```python
from build123d import *

# Parameters (mm, degrees)
SKETCH1_R           = 3.175
BOSS_EXTRUDE1_DEPTH = 25.4
SKETCH2_W           = 5.08
SKETCH2_H           = 2.9464
CUT_EXTRUDE1_DEPTH  = 9.144
BOSS_EXTRUDE2_START = 0.508
SKETCH3_R           = 3.175
BOSS_EXTRUDE2_DEPTH = 0.508
SKETCH4_R           = 2.667
SKETCH4_W           = 5.08
SKETCH4_H           = 2.921
CUT_EXTRUDE2_DEPTH  = 1.524


with BuildPart() as part:
    # Sketch1 → Boss-Extrude1 (new body)
    with BuildSketch(Plane(origin=(0, 0, 0), x_dir=(1, 0, 0), z_dir=(0, 1, 0))):
        with Locations(Location((0, 0, 0), (0, 0, 270))):
            Circle(SKETCH1_R)
    extrude(amount=BOSS_EXTRUDE1_DEPTH)

    # Sketch2 → Cut-Extrude1 (cut)
    with BuildSketch(Plane.XZ):
        Rectangle(SKETCH2_W, SKETCH2_H)
    extrude(amount=-CUT_EXTRUDE1_DEPTH, mode=Mode.SUBTRACT)

    # Sketch3 → Boss-Extrude2 (add)
    with BuildSketch(Plane.XZ.offset(BOSS_EXTRUDE2_START)):
        with Locations(Location((0, 0, 0), (0, 0, 270))):
            Circle(SKETCH3_R)
    extrude(amount=-BOSS_EXTRUDE2_DEPTH)

    # Sketch4 → Cut-Extrude2 (cut)
    with BuildSketch(Plane.XZ.offset(0.508)):
        Circle(SKETCH4_R)
        Rectangle(SKETCH4_W, SKETCH4_H)
    extrude(amount=-CUT_EXTRUDE2_DEPTH, mode=Mode.SUBTRACT)


solid = part.part
```
Build history of the part. All positions in model axes, mm. A direction names the side the tool comes from. Coordinates: 2 decimals unless noted, no trailing zeros. Order: outer loops, then holes, each group sorted by start corner. A loop starts at its lowest first (then second) coordinate and runs counter-clockwise, first axis right, second up. Notation, with made-up numbers: (-26.5, 68) -> (-14.5, 68) arc R11 ccw to (-14.5, 77) -> close; hole circle Ø8 at (-30.5, 81). An arc over 180 degrees is marked (long way). Answer in a Markdown table with one row per item. Add a question column.
Q1. Drop flat-ended pins along their axis: pin 1 (1.3 mm diameter, centred on x = 1, z = -2, fed in from -Y); pin 2 (0.9 mm diameter, centred on x = -1, z = -0.5, fed in from -Y); pin 3 (0.5 mm diameter, centred on y = 0.5, z = -1, fed in from -X); pin 4 (0.6 mm diameter, centred on y = 0, z = 1, fed in from +X). Give the stop position or say it passes through.
Q2. Mould opens along Y. For faces 3 (the face through (0, 1.016, -2)), 4 (the face through (0, 25.4, 0)) say: +Y half, -Y half, draft (parallel to the pull), parting line (faces both ways), or undercut.
Q3. Which spindle directions (+Z, -Z, +X, -X, +Y, -Y) get a long thin tool onto all of the face, cutting with end or side? Do faces 1 (the face through (2.667, 0.243, -0.012)), 2 (the face through (-2, -0.508, 2)). Say none if no direction does.
Q4. Wall check: line 1 along X through (y, z) = (3.5, 0) (3 decimals); line 2 along Y through (x, z) = (1.5, 0.75); line 3 along X through (y, z) = (9, -0.75). Give the ranges that are in metal, low to high. Write a range as [from, to].
Q5. Band-saw the part on B-B, the plane z = 0. List the corners of the cut face in (x, y) (3 decimals), then the cut area to 3 significant figures.
Q6. Band-saw the part on C-C, the plane x = 0. List the corners of the cut face in (y, z) (3 decimals), then the cut area to 3 significant figures.
Q7. Band-saw the part on A-A, the plane y = 2.25. List the corners of the cut face in (x, z) (3 decimals), then the cut area to 3 significant figures.
Q8. Band-saw the part on D-D, the plane y = 20. List the corners of the cut face in (x, z) (3 decimals), then the cut area to 3 significant figures.
Answers follow:
| question | item | result |
|---|---|---|
| 1 | pin 1 | y = -0.51 |
| 1 | pin 2 | y = 9.14 |
| 1 | pin 3 | x = -3.09 |
| 1 | pin 4 | x = 3.1 |
| 2 | face 3 | -Y half |
| 2 | face 4 | +Y half |
| 3 | face 1 | -Y |
| 3 | face 2 | +Z, -Z, +X, -X, -Y |
| 4 | line 1 | [-3.175, -2.54], [2.54, 3.175] |
| 4 | line 2 | [9.14, 25.4] |
| 4 | line 3 | [-3.09, -2.54], [2.54, 3.09] |
| 5 | outline | (-3.175, -0.508) -> (-2.667, -0.508) -> (-2.667, 1.016) -> (-2.54, 1.016) -> (-2.54, 9.144) -> (2.54, 9.144) -> (2.54, 1.016) -> (2.667, 1.016) -> (2.667, -0.508) -> (3.175, -0.508) -> (3.175, 25.4) -> (-3.175, 25.4) -> close |
| 5 | area | 115 mm^2 |
| 6 | outline | (-0.508, -3.175) -> (25.4, -3.175) -> (25.4, 3.175) -> (-0.508, 3.175) -> (-0.508, 2.667) -> (1.016, 2.667) -> (1.016, 1.473) -> (9.144, 1.473) -> (9.144, -1.473) -> (1.016, -1.473) -> (1.016, -2.667) -> (-0.508, -2.667) -> close |
| 6 | area | 132 mm^2 |
| 7 | outline | circle Ø6.35 at (0, 0); hole (-2.54, -1.473) -> (2.54, -1.473) -> (2.54, 1.473) -> (-2.54, 1.473) -> close |
| 7 | area | 16.7 mm^2 |
| 8 | outline | circle Ø6.35 at (0, 0) |
| 8 | area | 31.7 mm^2 |
